Verification items for the finished model (mm, model axes). A direction names the side the tool comes from. Round coordinates to 2 decimals unless told otherwise and drop trailing zeros. Order: outer loops, then holes, each group sorted by start corner. A loop starts at its lowest first (then second) coordinate and runs counter-clockwise, first axis right, second up. Notation, with made-up numbers: M -32,18.5 L -2,18.5 A19 cw -2,36.5 Z; hole C 2.5,36.25 d1. An arc over 180 degrees is marked long. Return JSON: item names as keys, results as strings. Group by question number.
from build123d import *

# Parameters (mm, degrees)
CUT_EXTRUDE_2_DEPTH    = 15
MM_CLEARANCE_1_D       = 12.1
MM_CLEARANCE_1_DEPTH   = 12
MM_CLEARANCE_1_TIP     = 3.635206745
HOLE_WIZARD_M4_3_D     = 3.3
HOLE_WIZARD_M4_3_DEPTH = 25
HOLE_WIZARD_M4_3_TIP   = 0.991420021


with BuildPart() as part:
    # 草图2 → 旋转1 (revolve)
    with BuildSketch(Plane.XY):
        Polygon((554.440585902, 10), (544.440585902, 10), (544.440585902, 25), (-25.559414098, 25), (-25.559414098, 10), (-35.559414098, 10), (-35.559414098, 8.5), (-45.559414098, 8.5), (-45.559414098, 7), (-65.559414098, 7), (-65.559414098, 0), (-51.631049649, 0), (574.440585902, 0), (574.440585902, 8.5), (554.440585902, 8.5), align=None)
    revolve(axis=Axis((-62.705882353, 0, 0), (1, 0, 0)))

    # 草图4 → 切除-拉伸2 (cut)
    with BuildSketch(Plane.ZY.offset(65.559414098)):
        with BuildLine():
            Line((-8, 6), (8, 6))
            ThreePointArc((8, 6), (0, 10), (-8, 6))
        make_face()
    extrude(amount=-CUT_EXTRUDE_2_DEPTH, mode=Mode.SUBTRACT)

    # 大小mm Clearance 暗销孔1
    with Locations(Plane(origin=(574.440585902, 0, 0), x_dir=(0, 0, -1), z_dir=(1, 0, 0))):
        with Locations((0, 0)):
            Hole(MM_CLEARANCE_1_D / 2, depth=MM_CLEARANCE_1_DEPTH)
            with Locations((0, 0, -(MM_CLEARANCE_1_DEPTH + MM_CLEARANCE_1_TIP / 2))):  # 118° drill point
                Cone(0, MM_CLEARANCE_1_D / 2, MM_CLEARANCE_1_TIP, mode=Mode.SUBTRACT)

    # M4 螺纹孔3
    with Locations(Plane(origin=(0, 8.5, 0), x_dir=(1, 0, 0), z_dir=(0, 1, 0))):
        with Locations((569.440585902, 0)):
            Hole(HOLE_WIZARD_M4_3_D / 2, depth=HOLE_WIZARD_M4_3_DEPTH)
            with Locations((0, 0, -(HOLE_WIZARD_M4_3_DEPTH + HOLE_WIZARD_M4_3_TIP / 2))):  # 118° drill point
                Cone(0, HOLE_WIZARD_M4_3_D / 2, HOLE_WIZARD_M4_3_TIP, mode=Mode.SUBTRACT)


solid = part.part
1. Cross-section at B-B (y = -16). Enter the section's corners in (x, z).
2. Access from +Z, -Z, +X, -X, +Y, -Y to the whole of each face (thin tool, end or side, straight path). Record for faces 1 (the face through (255.451, 23.846, 7.509)), 2 (the face through (554.441, 4.5, -7.4)), 3 (the face through (-56, -7, 0)).
3. Go/stop test with flat-tipped pins: pin 1 (1 mm diameter, centred on y = 0.5, z = 17.5, fed in from +X); pin 2 (2 mm diameter, centred on x = 569.44, z = 0, fed in from -Y); pin 3 (2 mm diameter, centred on x = 418.5, y = -18, fed in from -Z); pin 4 (3 mm diameter, centred on x = 297.5, z = 6, fed in from +Y). Record where each tip stops, or that it passes through.
4. Cross-section at C-C (y = 15.5). Enter the section's corners in (x, z), plus the area to 3 significant figures.
5. Thickness scan on line 1 along X through (y, z) = (-17, 14.5); line 2 along Z through (x, y) = (568.5, 0); line 3 along Y through (x, z) = (308, -2.5). Record the ranges inside material, lowest first. Write a range as from..to.
6. Draft check along Z on faces 4 (the face through (559.44, -1.03, 0.23)), 5 (the face through (564.3, 8.11, 2.55)), 6 (the face through (544.441, 0, -11)). Enter one of: +Z half, -Z half, draft (parallel to the pull), parting line (faces both ways), or undercut.
7. Cross-section at A-A (x = 441). Enter the section's corners in (y, z), plus the area to 3 significant figures.
Computed:
{
 "1": {"outline": "M -25.56,-19.21 L 544.44,-19.21 L 544.44,19.21 L -25.56,19.21 Z"},
 "2": {"face 1": "+X, -X", "face 2": "+X", "face 3": "-X"},
 "3": {"pin 1": "stops at x = 544.44", "pin 2": "passes through", "pin 3": "stops at z = -18.33", "pin 4": "stops at y = 24.59"},
 "4": {"outline": "M -25.56,-19.62 L 544.44,-19.62 L 544.44,19.62 L -25.56,19.62 Z", "area": "22,400 mm²"},
 "5": {"line 1": "x = -25.56..544.44", "line 2": "z = -8.5..-6.05, 6.05..8.5", "line 3": "y = -24.87..24.87"},
 "6": {"face 4": "undercut", "face 5": "parting line", "face 6": "draft"},
 "7": {"outline": "C 0,0 d50", "area": "1,960 mm²"}
}
